```python
from build123d import *

# Parameters (mm, degrees)
SKETCH_1_W          = 80
SKETCH_1_H          = 30
EXTRUDE_1_DEPTH     = 33.2
SKETCH_2_R          = 4
CUT_EXTRUDE_1_DEPTH = 34.2
CUT_EXTRUDE_4_DEPTH = 30
CUT_EXTRUDE_5_DEPTH = 30


with BuildPart() as part:
    # Эскиз1 → Бобышка-Вытянуть1 (new body)
    with BuildSketch(Plane(origin=(0, 0, 0), x_dir=(1, 0, 0), z_dir=(0, 1, 0))):
        Rectangle(SKETCH_1_W, SKETCH_1_H)
    extrude(amount=EXTRUDE_1_DEPTH)

    # Эскиз2 → Вырез-Вытянуть1 (cut, through all)
    with BuildSketch(Plane(origin=(0, 33.2, 0), x_dir=(1, 0, 0), z_dir=(0, 1, 0))):
        with Locations(Location((0, 0, 0), (0, 0, 270))):  # turned: the seam where the file's is
            Circle(SKETCH_2_R)
    extrude(amount=-CUT_EXTRUDE_1_DEPTH, mode=Mode.SUBTRACT)

    # Эскиз5 → Вырез-Вытянуть4 (cut)
    with BuildSketch(Plane.ZY.offset(40)):
        Polygon((-11.015265685, 14.014671802), (-4.458832066, 6.201018482), (11.015265685, 19.185328198), (4.458832066, 26.998981518), align=None)
    extrude(amount=-CUT_EXTRUDE_4_DEPTH, mode=Mode.SUBTRACT)

    # Эскиз6 → Вырез-Вытянуть5 (cut)
    with BuildSketch(Plane(origin=(40, 0, 0), x_dir=(0, 0, -1), z_dir=(1, 0, 0))):
        Polygon((11.015265685, 14.014671802), (4.458832066, 6.201018482), (-11.015265685, 19.185328198), (-4.458832066, 26.998981518), align=None)
    extrude(amount=-CUT_EXTRUDE_5_DEPTH, mode=Mode.SUBTRACT)


solid = part.part
```
Design review of the part built by this model. Coordinates are the model's own, in mm. A direction names the side the tool comes from. Coordinates: 2 decimals unless noted, no trailing zeros. Loops run counter-clockwise (first coordinate to the right, second up) from the corner with the lowest first, then second, coordinate; pieces in that order, holes last. Notation, with made-up numbers: M 26,21 L 33,21 A18 cw 33,30 Z; hole C 87.25,60.25 d6. An arc over 180 degrees is marked long. One line per question, with ' | ' between items.
(1) Machinability: for faces 4 (the face through (25.21, 20.6, -3.17)), 5 (the face through (-1, 16, -15)), 6 (the face through (-25.21, 23.04, 7.78)), which of the approach directions +Z, -Z, +X, -X, +Y, -Y give a long, thin tool a straight path to every point of the face, cutting with its end or side? Answer none if there is none.
Filled in:
face 4: +X | face 5: -Z, +X, -X, +Y, -Y | face 6: -X
(2) We need section C-C (x = 0). Give the boundary of the cut face in (y, z).
Filled in:
outline: M 0,-15 L 33.2,-15 L 33.2,-4 L 0,-4 Z; M 0,4 L 33.2,4 L 33.2,15 L 0,15 Z
(3) We need section D-D (y = 29.5). Give the boundary of the cut face in (x, z), and give its area (3 significant figures).
Filled in:
outline: M -40,-15 L 40,-15 L 40,15 L -40,15 Z; hole C 0,0 d8 | area: 2,350 mm^2
(4) Wall thickness on probe 1 along X at (y, z) = (26, 0); probe 2 along Y at (x, z) = (-17, -1.5); probe 3 along Z at (x, y) = (-13, 20.5): over which ranges is each line inside the solid? List them lowest first.
Filled in:
probe 1: x = -40 to -4, 4 to 40 | probe 2: y = 0 to 8.68, 22 to 33.2 | probe 3: z = -15 to -3.29, 9.91 to 15
(5) For pin 1 Ø10.5 at (y, z) = (19, 4) entering from -X; pin 2 Ø5 at (y, z) = (11, -4.5) entering from -X, all flat-tipped, find the tip position at first contact; note any pin that passes through.
Filled in:
pin 1: stops at x = -40 | pin 2: stops at x = -10
(6) We need section B-B (z = 0). Give the boundary of the cut face in (x, y), and give its area (3 significant figures).
Filled in:
outline: M -40,0 L -4,0 L -4,33.2 L -40,33.2 L -40,23.26 L -10,23.26 L -10,9.94 L -40,9.94 Z; M 4,0 L 40,0 L 40,9.94 L 10,9.94 L 10,23.26 L 40,23.26 L 40,33.2 L 4,33.2 Z | area: 1,590 mm^2
(7) Draft analysis for pull direction Z (two halves, no side actions). For faces 1 (the face through (40, 13, 4)), 2 (the face through (-25.21, 10.16, -7.78)), 3 (the face through (-1, 16, 15)), state which applies: released by +Z, released by -Z, zero draft, split by the parting line, or undercut.
Filled in:
face 1: zero draft | face 2: undercut | face 3: released by +Z
(8) We need section A-A (x = -11.5). Give the boundary of the cut face in (y, z), and give its area (3 significant figures).
Filled in:
outline: M 0,-15 L 33.2,-15 L 33.2,15 L 0,15 Z; hole M 6.2,-4.46 L 14.01,-11.02 L 27,4.46 L 19.19,11.02 Z | area: 790 mm^2
